Geometry check sheet. Reference: the model listing, model coordinates, mm. A direction names the side the tool comes from. Give positions to 0.01 mm unless a question says otherwise; leave off trailing zeros. Order: outer loops, then holes, each group sorted by start corner. A loop starts at its lowest first (then second) coordinate and runs counter-clockwise, first axis right, second up. Notation, with made-up numbers: M -2,12 L 2,12 A13 ccw 2,24 Z; hole C 16.25,20 d7. An arc over 180 degrees is marked long. Answer as CSV lines item,"result". Start each with the question number.
Q1. Mould release check, pull along X, two halves, no side actions. Record for faces 1 (the flat face through (30.44, 1.46, 6.3)), 2 (the flat face through (18, 2, 16)): +X half, -X half, draft (parallel to the pull), parting line (faces both ways), or undercut.
Q2. Section check B-B, the plane x = 18. Record the boundary of the cut face in (y, z).
Q3. Set-up check for faces 3 (the flat face through (18, 2.5, 19)), 4 (the flat face through (18, -1, 16)), 5 (the flat face through (18, 0, 18.5)), 6 (the flat face through (5.61, 1.46, 6.48)), 7 (the flat face through (18, 3, 22)): record each of +Z, -Z, +X, -X, +Y, -Y from which the full face is reachable in a straight line by a thin tool's end or side.
Q4. Section check C-C, the plane z = 7.25. Record the boundary of the cut face in (x, y), then the cut area to 3 significant figures.
Q5. Go/stop test with flat-tipped pins: pin 1 (3 mm diameter, centred on x = 5, z = 6, fed in from -Y); pin 2 (6.5 mm diameter, centred on x = 14, z = 10, fed in from -Y); pin 3 (1.5 mm diameter, centred on y = 2, z = 11, fed in from +X); pin 4 (5 mm diameter, centred on x = 9.5, z = 19, fed in from -Y). Record where each tip stops, or that it passes through.
Q6. Section check D-D, the plane y = 1.5. Record the boundary of the cut face in (x, z), then the cut area to 3 significant figures.
Q7. Thickness scan on line 1 (Y direction, x = 30, z = 20.5); line 2 (X direction, y = -2, z = 7); line 3 (X direction, y = -0.5, z = 11.5). Record the ranges inside material, lowest first.
Q8. Section check A-A, the plane z = 16.5. Record the boundary of the cut face in (x, y), then the cut area to 3 significant figures.
```python
from build123d import *

# Parameters (mm, degrees)
F1_DEPTH = 22
F2_W     = 44
F2_H     = 2
F3_DEPTH = 6
F5_DEPTH = 5
F6_W     = 12
F6_H     = 3.5
F7_DEPTH = 3.5
F8_R     = 3


with BuildPart() as f1:
    # F0 (on Top) → F1 (new body)
    with BuildSketch(Plane.XY):
        with BuildLine():
            ThreePointArc((3.872983, -1), (3.968119, -0.504017), (4, 0))
            ThreePointArc((4, 0), (2.828427, 2.828427), (0, 4))
            ThreePointArc((0, 4), (-3.162278, -2.44949), (3.872983, -1))
        make_face()
        with BuildLine():
            ThreePointArc((0, 4), (2.828427, 2.828427), (4, 0))
            ThreePointArc((4, 0), (3.968119, -0.504017), (3.872983, -1))
            Line((3.872983, -1), (32.127017, -1))
            ThreePointArc((32.127017, -1), (32.837722, 2.44949), (36, 4))
            Line((36, 4), (0, 4))
        make_face()
        with BuildLine():
            ThreePointArc((40, 0), (38.828427, 2.828427), (36, 4))
            ThreePointArc((36, 4), (32.837722, 2.44949), (32.127017, -1))
            ThreePointArc((32.127017, -1), (36.504017, -3.968119), (40, 0))
        make_face()
    extrude(amount=F1_DEPTH)

    # F2 (on face) → F3 (cut)
    with BuildSketch(Plane.XY.offset(22)):
        with Locations((18, 1.5)):
            Rectangle(F2_W, F2_H)
    extrude(amount=-F3_DEPTH, mode=Mode.SUBTRACT)

    # F4 (on face) → F5 (cut, through all)
    with BuildSketch(Plane.XZ.offset(1)):
        Polygon((7.892221, 15), (3.872983, 0), (32.127017, 0), (28.107779, 15), (18, 15), align=None)
    extrude(amount=-F5_DEPTH, mode=Mode.SUBTRACT)

    # F6 (on face) → F7 (cut)
    with BuildSketch(Plane.XZ.offset(1)):
        with Locations((18, 20.25)):
            Rectangle(F6_W, F6_H)
    extrude(amount=-F7_DEPTH, mode=Mode.SUBTRACT)

    # F8
    f8_edges = [f1.edges().sort_by_distance(p)[0] for p in [
        (7.892221, 1.5, 15),
        (28.107779, 1.5, 15),
    ]]
    fillet(f8_edges, radius=F8_R)


solid = f1.part
```
Answer block:
1,face 1,"undercut"
1,face 2,"draft"
2,outline,"M -1,15 L 4,15 L 4,22 L 2.5,22 L 2.5,16 L 0.5,16 L 0.5,18.5 L -1,18.5 Z"
3,face 3,"+Z, +X, -X"
3,face 4,"+Z, -Z, -Y"
3,face 5,"+Z, -Y"
3,face 6,"-Z, +Y, -Y"
3,face 7,"+Z, +X, -X, +Y, -Y"
4,outline,"M 0,4 A4 ccw long 3.87,-1 L 5.82,-1 L 5.82,4 Z; M 30.18,-1 L 32.13,-1 A4 ccw long 36,4 L 30.18,4 Z"
4,area,"126 mm2"
5,pin 1,"stops at y = -1.94"
5,pin 2,"passes through"
5,pin 3,"stops at x = 39.8"
5,pin 4,"stops at y = -1"
6,outline,"M -3.71,0 L 3.87,0 L 7.3,12.78 A3 cw 10.19,15 L 25.81,15 A3 cw 28.7,12.78 L 32.13,0 L 39.71,0 L 39.71,16 L -3.71,16 Z"
6,area,"333 mm2"
7,line 1,"y = -1 to 0.5, 2.5 to 4"
7,line 2,"x = -3.46 to 3.46, 32.54 to 39.46"
7,line 3,"x = -3.97 to 6.95, 29.05 to 39.97"
8,outline,"M -3.97,0.5 A4 ccw 3.87,-1 L 32.13,-1 A4 ccw 39.97,0.5 Z; M -3.12,2.5 L 39.12,2.5 A4 ccw 36,4 L 0,4 A4 ccw Z"
8,area,"161 mm2"
